Source: CAD feature listing. Evaluate the final solid. Frame: model axes, mm. A direction names the side the tool comes from. Round coordinates to 2 decimals unless told otherwise and drop trailing zeros. Order: outer loops, then holes, each group sorted by start corner. A loop starts at its lowest first (then second) coordinate and runs counter-clockwise, first axis right, second up. Notation, with made-up numbers: (-35, 54) -> (3, 54) arc R15 ccw to (3, 81) -> close; hole circle Ø6 at (57, 29). An arc over 180 degrees is marked (long way). One line per item, written item: value. Start each with the question number.
1) Pin query (flat end, axial travel): P1, Ø7, axis at x = 132, z = 18.5, coming from the -Y side; P2, Ø1, axis at x = 146, y = 292.5, coming from the +Z side; P3, Ø4, axis at y = 276, z = 110.5, coming from the +X side; P4, Ø6, axis at x = 141.5, z = 95, coming from the -Y side. Return the tip coordinate at first contact, or that it passes through.
2) Section B-B (z = 55). Return the cut outline in (x, y), and give its area (3 significant figures).
3) Ray query, L1, parallel to Z at x = 136, y = 247; L2, parallel to X at y = 298.5, z = 113.5 (3 decimals); L3, parallel to Z at x = 110, y = 265.5. Return the intervals inside material, ascending.
4) Section C-C (z = 182). Return the cut outline in (x, y), and give its area (3 significant figures).
5) Reachability of faces 1 (the face through (142.58, 259.87, 163.74)), 2 (the face through (129, 310.898, 30)), 3 (the face through (139.43, 303.49, 163.74)) from +Z, -Z, +X, -X, +Y, -Y: full face, straight path, thin tool, end or side. Return the list, or none.
6) Mould query, pull axis Z, two halves, no side actions, for faces 4 (the face through (137.3, 282.1, 61.016)), 5 (the face through (99.675, 246.409, 149.796)), 6 (the face through (125.198, 254.626, 163.74)). Classes: pulls with the +Z half, pulls with the -Z half, needs draft (parallel to the pull), parting line crosses it, or undercut.
7) Section A-A (z = 129). Return the cut outline in (x, y).
```python
from build123d import *

# Parameters (mm, degrees)
SKETCH1_W           = 24.092408
SKETCH1_H           = 58.498994
BOSS_EXTRUDE1_DEPTH = 61.016388
SKETCH2_R           = 6.346800124
BOSS_EXTRUDE2_DEPTH = 83.73364
BOSS_EXTRUDE3_DEPTH = 10.235946
BOSS_EXTRUDE3_DRAFT = -10
BOSS_EXTRUDE4_DEPTH = 22.011894
CHAMFER1_SIZE       = 4.256024


with BuildPart() as part:
    # Sketch1 → Boss-Extrude1 (new body)
    with BuildSketch(Plane.XY):
        with Locations((129.44221, 281.648027)):
            Rectangle(SKETCH1_W, SKETCH1_H)
    extrude(amount=BOSS_EXTRUDE1_DEPTH)

    # Sketch2 → Boss-Extrude2 (add)
    with BuildSketch(Plane.XY.offset(61.016388)):
        with Locations((128.797304, 299.288048124)):
            Circle(SKETCH2_R)
        Polygon((118.62689, 289.014154), (121.536714, 291.906706), (133.935216, 292.005766), (136.89203, 289.161982), (137.15365, 259.165852), (134.240778, 256.272792), (121.831608, 256.171192), (118.88851, 259.018278), align=None)
    extrude(amount=BOSS_EXTRUDE2_DEPTH)


with BuildPart() as boss_extrude3_tool:
    # Sketch3 → Boss-Extrude3 (with draft: the straight prism first)
    with BuildSketch(Plane.XY.offset(144.750028)):
        Polygon((92.973398, 306.72786), (96.953832, 249.578876), (103.696262, 244.488716), (148.240242, 247.626124), (154.211274, 253.612142), (150.230586, 310.760872), (143.488156, 315.851286), (98.94443, 312.713624), align=None)
    extrude(amount=BOSS_EXTRUDE3_DEPTH)
    # Boss-Extrude3: the draft: its side faces are tilted about the plane it starts from
    boss_extrude3_sides = [boss_extrude3_tool.faces().sort_by_distance(p)[0] for p in [
        (94.963615, 278.153368, 149.868001),
        (100.325047, 247.033796, 149.868001),
        (125.968252, 246.05742, 149.868001),
        (151.225758, 250.619133, 149.868001),
        (152.22093, 282.186507, 149.868001),
        (146.859371, 313.306079, 149.868001),
        (121.216293, 314.282455, 149.868001),
        (95.958914, 309.720742, 149.868001),
    ]]
    draft(boss_extrude3_sides, Plane.XY.offset(144.750028), BOSS_EXTRUDE3_DRAFT)


with BuildPart() as part_1:
    add(part.part)

    # Boss-Extrude3: add boss_extrude3_tool
    add(boss_extrude3_tool.part)

    # Sketch4 → Boss-Extrude4 (add)
    with BuildSketch(Plane.XY.offset(154.985974)):
        Polygon((100.368862, 296.721784), (107.41025, 305.1429), (135.417814, 307.115718), (143.557752, 299.763942), (146.04746, 264.019538), (139.006072, 255.598422), (110.998508, 253.625604), (102.858316, 260.97738), align=None)
    extrude(amount=BOSS_EXTRUDE4_DEPTH)

    # Chamfer1
    chamfer1_edges = [part_1.edges().sort_by_distance(p)[0] for p in [
        (101.613589, 278.849582, 176.997868),
        (106.928412, 257.301492, 176.997868),
        (125.00229, 254.612013, 176.997868),
        (142.526766, 259.80898, 176.997868),
        (144.802606, 281.89174, 176.997868),
        (139.487783, 303.43983, 176.997868),
        (121.414032, 306.129309, 176.997868),
        (103.889556, 300.932342, 176.997868),
    ]]
    chamfer(chamfer1_edges, length=CHAMFER1_SIZE)

    # Sketch6 → Revolve1 (revolve)
    with BuildSketch(Plane(origin=(123.208151271, 0, 0), x_dir=(0, 0, -1), z_dir=(1, 0, 0)), mode=Mode.PRIVATE) as revolve1_sk:
        with BuildLine():
            Line((-176.997868, 280.370660315), (-176.997868, 289.089464315))
            Line((-176.997868, 289.089464315), (-188.349382, 289.089464315))
            ThreePointArc((-188.349382, 289.089464315), (-209.048874501, 298.213625605), (-222.953834, 280.370660315))
            Line((-222.953834, 280.370660315), (-176.997868, 280.370660315))
        make_face()
    revolve(revolve1_sk.sketch.rotate(Axis((123.208151271, 280.370660315, 176.997868), (0, 0, 1)), 90), axis=Axis((123.208151271, 280.370660315, 176.997868), (0, 0, 1)))


solid = part_1.part
```
Findings:
1. P1: y = 252.4
1. P2: z = 154.99
1. P3: x = 137.02
1. P4: through
2. outline: (117.4, 252.4) -> (141.49, 252.4) -> (141.49, 310.9) -> (117.4, 310.9) -> close
2. area: 1,410 mm2
3. L1: 144.75 to 154.99
3. L2: 122.5 to 135.095
3. L3: 144.75 to 177
4. outline: circle Ø17.44 at (123.21, 280.37)
4. area: 239 mm2
5. face 1: +Z, +X, -Y
5. face 2: -Z, +X, -X, +Y
5. face 3: +Z, +X, +Y
6. face 4: undercut
6. face 5: pulls with the -Z half
6. face 6: needs draft
7. outline: (118.63, 289.01) -> (118.89, 259.02) -> (121.83, 256.17) -> (134.24, 256.27) -> (137.15, 259.17) -> (136.89, 289.16) -> (133.94, 292.01) -> (121.54, 291.91) -> close; circle Ø12.69 at (128.8, 299.29)
